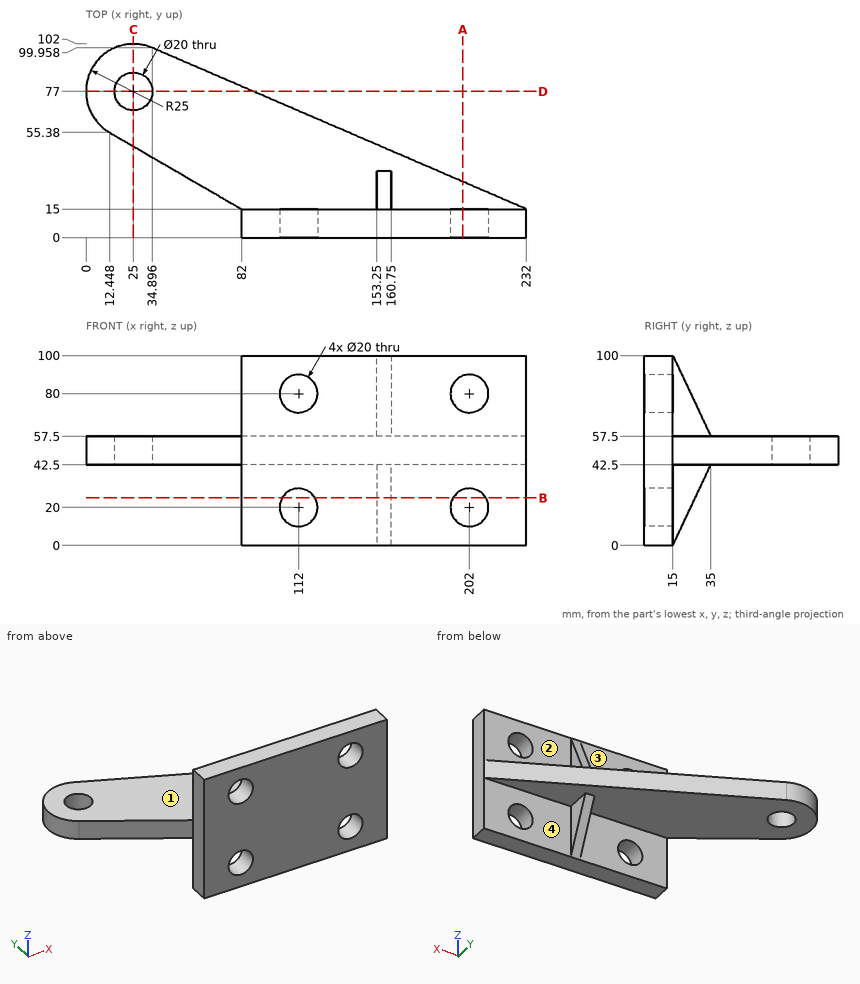
Print and shaded views of the part. All mm, measured from the part's lowest x, y and z. A direction names the side the tool comes from. Round coordinates to 2 decimals unless told otherwise and drop trailing zeros. Loops run counter-clockwise (first coordinate to the right, second up) from the corner with the lowest first, then second, coordinate; pieces in that order, holes last. Notation, with made-up numbers: M 27,6 L 32,6 A18 cw 32,25 Z; hole C -20,-36.5 d6. An arc over 180 degrees is marked long. One line per question, with ' | ' between items.
1) Drill centre lines: line 1 along X through (y, z) = (11, 20); line 2 along Z through (x, y) = (112, 9); line 3 along Z through (x, y) = (93.5, 39). Where is each one in solid material? Low to high.
Solved:
line 1: x = 82 to 102, 122 to 192, 212 to 232 | line 2: z = 0 to 10, 30 to 70, 90 to 100 | line 3: z = 42.5 to 57.5
2) Band-saw the part on D-D (y = 77). Give the cut face in (x, z).
Solved:
outline: M 0,42.5 L 15,42.5 L 15,57.5 L 0,57.5 Z; M 35,42.5 L 88.16,42.5 L 88.16,57.5 L 35,57.5 Z
3) Flat gauge pins, fed straight in: pin 1 (22 mm diameter, centred on y = 25, z = 69, fed in from -X); pin 2 (6 mm diameter, centred on y = 26.5, z = 30, fed in from +X); pin 3 (10 mm diameter, centred on y = 77, z = 57, fed in from +X); pin 4 (12 mm diameter, centred on x = 25, y = 77, fed in from -Z). Where does each tip first touch, or does it go through?
Solved:
pin 1: stops at x = 82 | pin 2: stops at x = 160.75 | pin 3: stops at x = 99.76 | pin 4: passes through
4) Band-saw the part on C-C (x = 25). Give the cut face in (y, z).
Solved:
outline: M 48.09,42.5 L 67,42.5 L 67,57.5 L 48.09,57.5 Z; M 87,42.5 L 102,42.5 L 102,57.5 L 87,57.5 Z
5) Band-saw the part on A-A (x = 198.5). Give the cut face in (y, z).
Solved:
outline: M 0,0 L 15,0 L 15,10.63 L 0,10.63 Z; M 0,29.37 L 15,29.37 L 15,42.5 L 29.44,42.5 L 29.44,57.5 L 15,57.5 L 15,70.63 L 0,70.63 Z; M 0,89.37 L 15,89.37 L 15,100 L 0,100 Z
6) Band-saw the part on B-B (z = 25). Give the number of separate pieces and of enclosed holes in the cut face, then the cut area to 3 significant figures.
Solved:
separate pieces: 3 | enclosed holes: 0 | area: 1,820 mm²
7) 3-axis set-ups, long thin cutter, end or side, ignore diameter. For the marked faces 1, 2, 3 and 4: which of +Z, -Z, +X, -X, +Y, -Y reach the whole face in a straight line?
Solved:
face 1: +Z, +Y | face 2: +Z, +X, +Y | face 3: +Z, -X, +Y | face 4: -Z, +X, +Y
